The figure shows three views and two pictorial views of one solid part (mm, origin at its lowest corner). Answer the questions. Coordinates: 2 decimals unless noted, no trailing zeros. Write each loop counter-clockwise with the first axis right and the second up, starting at its lowest first coordinate (ties: lowest second). Pieces come first, ordered by that corner, then holes.
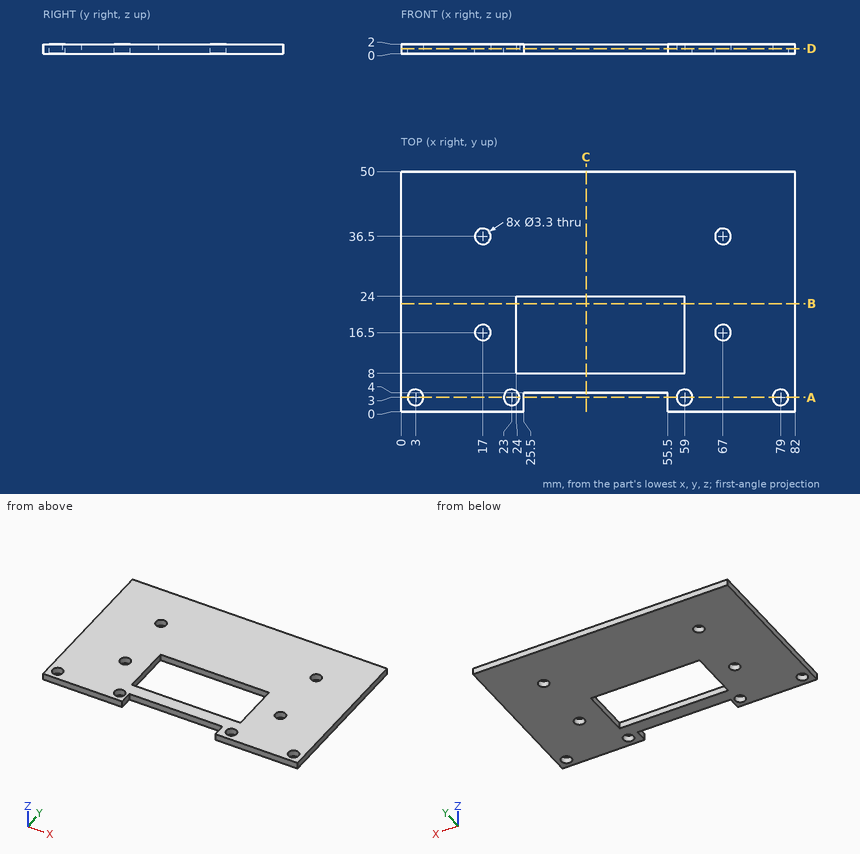
1. Section D-D on z = 1.05 is taken. State how many separate pieces and enclosed holes the cut face has, then the cut area to 3 significant figures.
Results found:
separate pieces: 1
enclosed holes: 9
area: 3,350 mm2
2. Section A-A on y = 3 is taken. Give the vertices of the cut face in (x, z).
Results found:
outline: (0, 0) - (1.35, 0) - (1.35, 2) - (0, 2) - close; (4.65, 0) - (21.35, 0) - (21.35, 2) - (4.65, 2) - close; (24.65, 0) - (25.5, 0) - (25.5, 2) - (24.65, 2) - close; (55.5, 0) - (57.35, 0) - (57.35, 2) - (55.5, 2) - close; (60.65, 0) - (77.35, 0) - (77.35, 2) - (60.65, 2) - close; (80.65, 0) - (82, 0) - (82, 2) - (80.65, 2) - close
3. Find the intervals of material crossed by L1, parallel to Y at x = 48, z = 1; L2, parallel to X at y = 23.5, z = 0.75; L3, parallel to Y at x = 17, z = 1.3, in increasing order.
Results found:
L1: y = 4 to 8, 24 to 50
L2: x = 0 to 24, 59 to 82
L3: y = 0 to 14.85, 18.15 to 34.85, 38.15 to 50
4. Section C-C on x = 38.5 is taken. Give the vertices of the cut face in (y, z), then the cut area to 3 significant figures.
Results found:
outline: (4, 0) - (8, 0) - (8, 2) - (4, 2) - close; (24, 0) - (50, 0) - (50, 2) - (24, 2) - close
area: 60.0 mm2
5. Section B-B on y = 22.5 is taken. Give the vertices of the cut face in (x, z), then the cut area to 3 significant figures.
Results found:
outline: (0, 0) - (24, 0) - (24, 2) - (0, 2) - close; (59, 0) - (82, 0) - (82, 2) - (59, 2) - close
area: 94.0 mm2
